The listing builds one solid part. Answer for the finished solid, in the listing's coordinates (mm). Face numbers are marked on the shaded views. Give positions to 0.01 mm unless a question says otherwise; leave off trailing zeros. Write each loop counter-clockwise with the first axis right and the second up, starting at its lowest first coordinate (ties: lowest second). Pieces come first, ordered by that corner, then holes. Notation, with made-up numbers: (3.5, 8.5) -> (41.5, 8.5) arc R25 ccw to (41.5, 22.5) -> close; hole circle Ø5 at (-20, 59.25). An arc over 180 degrees is marked (long way). Put each result on its own line as item: value. Start each with the question number.
1) A cutting plane is placed at A-A (y = 16). Write down the section's boundary in (x, z).
2) A cutting plane is placed at B-B (z = 3). Write down the section's boundary in (x, y), then the cut area to 3 significant figures.
3) A cutting plane is placed at C-C (x = 0). Write down the section's boundary in (y, z).
4) Find the intervals of material crossed by line 1 along Z through (x, y) = (8.5, 5.5); line 2 along Z through (x, y) = (7.5, 12.5); line 3 along X through (y, z) = (8.5, -3.75), in increasing order. Write a range as from..to.
5) Flat-ended cylindrical pins translate along their axes: pin 1 Ø5 at (x, z) = (-7.5, -1) entering from +Y (3 decimals); pin 2 Ø1 at (x, z) = (1.5, -10.5) entering from +Y; pin 3 Ø1.5 at (x, z) = (6, 0.5) entering from -Y; pin 4 Ø1.5 at (x, y) = (7, 27.5) entering from +Z. Find the tip coordinate at first contact, or state that the pin passes through.
6) For a pull along Z with two mould halves and no side action, classify the marked faces 1, 2 and 3 as released by +Z, released by -Z, zero draft, split by the parting line, or undercut.
from build123d import *

# Parameters (mm, degrees)
EXTRUDE_1_DEPTH     = 40
CUT_EXTRUDE_1_DEPTH = 40


with BuildPart() as part:
    # 草图1 → 凸台-拉伸1 (new body)
    with BuildSketch(Plane(origin=(0, 0, 0), x_dir=(1, 0, 0), z_dir=(0, 1, 0))):
        with BuildLine():
            Line((0, 19.95), (10, 19.95))
            Line((10, 19.95), (10, 14.95))
            Line((10, 14.95), (5, 9.947267065))
            Line((5, 9.947267065), (5, 8.660254038))
            ThreePointArc((5, 8.660254038), (0, -10), (-5, 8.660254038))
            Line((-5, 8.660254038), (-5, 9.947267065))
            Line((-5, 9.947267065), (-10, 14.95))
            Line((-10, 14.95), (-10, 19.95))
            Line((-10, 19.95), (0, 19.95))
        make_face()
    extrude(amount=EXTRUDE_1_DEPTH)

    # 草图3 → 切除-拉伸1 (cut)
    with BuildSketch(Plane.ZY.offset(10)):
        Polygon((10, 20), (-19.95, 40), (10, 40), align=None)
    extrude(amount=-CUT_EXTRUDE_1_DEPTH, mode=Mode.SUBTRACT)


solid = part.part
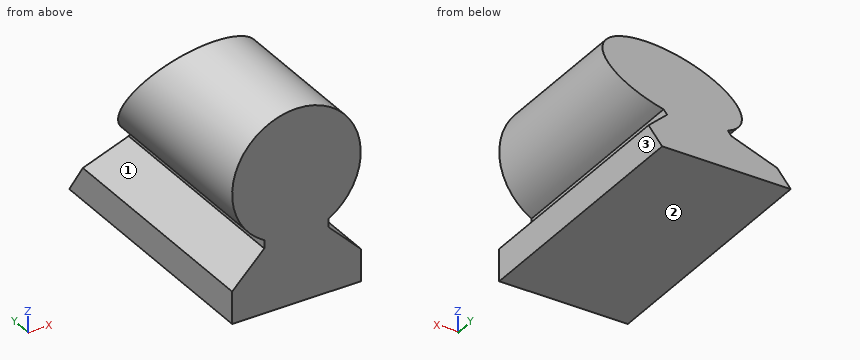
Reply:
1. outline: (-10, -19.95) -> (10, -19.95) -> (10, -14.95) -> (5, -9.95) -> (5, -8.66) arc R10 ccw (long way) to (-5, -8.66) -> (-5, -9.95) -> (-10, -14.95) -> close
2. outline: (-9.54, 0) -> (9.54, 0) -> (9.54, 24.67) -> (-9.54, 24.67) -> close
2. area: 471 mm2
3. outline: (0, -19.95) -> (40, -19.95) -> (20, 10) -> (0, 10) -> close
4. line 1: z = -19.95..-13.45, -5.27..5.27
4. line 2: z = -19.95..-12.45, -6.61..6.61
4. line 3: x = -9.27..9.27
5. pin 1: stops at y = 29.015
5. pin 2: stops at y = 34.02
5. pin 3: stops at y = 0
5. pin 4: stops at z = -0.11
6. face 1: undercut
6. face 2: released by -Z
6. face 3: zero draft
